Source: CAD feature listing. Evaluate the final solid. Frame: model axes, mm. Face numbers are marked on the shaded views. Give positions to 0.01 mm unless a question says otherwise; leave off trailing zeros. Loops run counter-clockwise (first coordinate to the right, second up) from the corner with the lowest first, then second, coordinate; pieces in that order, holes last.
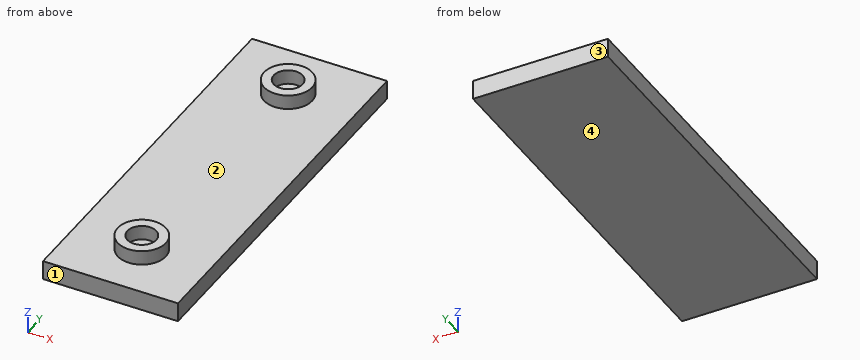
from build123d import *

# Parameters (mm, degrees)
F0_W          = 14
F0_H          = 2
F1_DEPTH      = 20
F1_DEPTH_BACK = 20
F2_R          = 2.5
F2_R_2        = 1.5
F3_DEPTH      = 1.5


with BuildPart() as f1:
    # F0 (on Front) → F1 (new body, two sides)
    with BuildSketch(Plane.XZ) as f1_sk:
        with Locations((0, 1)):
            Rectangle(F0_W, F0_H)
    extrude(amount=F1_DEPTH)
    extrude(f1_sk.sketch, amount=-F1_DEPTH_BACK)

    # F2 (on face) → F3 (join)
    with BuildSketch(Plane.XY.offset(2)):
        with Locations((0, 14)):
            Circle(F2_R)
        with Locations((0, 14)):
            Circle(F2_R_2, mode=Mode.SUBTRACT)
        with Locations((0, -14)):
            Circle(F2_R)
        with Locations((0, -14)):
            Circle(F2_R_2, mode=Mode.SUBTRACT)
    extrude(amount=F3_DEPTH)


solid = f1.part
1) Cut plane D-D (x = 2). Return loops of the section in (y, z), and give its area (3 significant figures).
Checks:
outline: (-20, 0) - (20, 0) - (20, 2) - (15.5, 2) - (15.5, 3.5) - (12.5, 3.5) - (12.5, 2) - (-12.5, 2) - (-12.5, 3.5) - (-15.5, 3.5) - (-15.5, 2) - (-20, 2) - close
area: 89.0 mm2
2) Cut plane A-A (x = 0). Return loops of the section in (y, z), and give its area (3 significant figures).
Checks:
outline: (-20, 0) - (20, 0) - (20, 2) - (16.5, 2) - (16.5, 3.5) - (15.5, 3.5) - (15.5, 2) - (12.5, 2) - (12.5, 3.5) - (11.5, 3.5) - (11.5, 2) - (-11.5, 2) - (-11.5, 3.5) - (-12.5, 3.5) - (-12.5, 2) - (-15.5, 2) - (-15.5, 3.5) - (-16.5, 3.5) - (-16.5, 2) - (-20, 2) - close
area: 86.0 mm2
3) Pull-direction query (Y, two-part tool) for the marked faces 1, 2, 3 and 4; classes: released by +Y, released by -Y, zero draft, split by the parting line, or undercut.
Checks:
face 1: released by -Y
face 2: undercut
face 3: released by +Y
face 4: zero draft
4) Contact query for a flat-ended pin moving along its axis: P1, Ø1.8, axis at x = 0, y = -14, coming from the +Z side. Output: stop coordinate, or through.
Checks:
P1: stops at z = 2
5) Ray query, probe 1 along Y at (x, z) = (0, 2.7); probe 2 along Z at (x, y) = (-4.5, -4). Return the intervals inside material, ascending.
Checks:
probe 1: y = -16.5 to -15.5, -12.5 to -11.5, 11.5 to 12.5, 15.5 to 16.5
probe 2: z = 0 to 2
6) Cut plane C-C (y = -14). Return loops of the section in (x, z), and give its area (3 significant figures).
Checks:
outline: (-7, 0) - (7, 0) - (7, 2) - (2.5, 2) - (2.5, 3.5) - (1.5, 3.5) - (1.5, 2) - (-1.5, 2) - (-1.5, 3.5) - (-2.5, 3.5) - (-2.5, 2) - (-7, 2) - close
area: 31.0 mm2
7) Cut plane B-B (z = 2.5). Return loops of the section in (x, y), and give its area (3 significant figures).
Checks:
outline: circle Ø5 at (0, -14); circle Ø5 at (0, 14); hole circle Ø3 at (0, -14); hole circle Ø3 at (0, 14)
area: 25.1 mm2
